```python
from build123d import *

# Parameters (mm, degrees)
F1_DEPTH = 30
F2_W     = 30
F2_H     = 30
F3_DEPTH = 1440
F4_W     = 1440
F4_H     = 1640
F5_DEPTH = 30
F7_DEPTH = 30


with BuildPart() as f1:
    # F0 (on Front) → F1 (new body)
    with BuildSketch(Plane.XZ):
        Polygon((0, 1700), (0, 0), (1500, 0), (1500, 1700), (0, 1900), align=None)
        Polygon((30, 1500), (30, 1670), (1470, 1670), (1470, 30), (30, 30), align=None, mode=Mode.SUBTRACT)
        Polygon((30, 1865.734508), (1273.008811, 1700), (30, 1700), align=None, mode=Mode.SUBTRACT)
    extrude(amount=F1_DEPTH)

    # F2 (on face) → F3 (join)
    with BuildSketch(Plane.XZ.offset(30)):
        with Locations((15, 15)):
            Rectangle(F2_W, F2_H)
        with Locations((1485, 15)):
            Rectangle(F2_W, F2_H)
        with Locations((15, 1685)):
            Rectangle(F2_W, F2_H)
        with Locations((1485, 1685)):
            Rectangle(F2_W, F2_H)
        with Locations((15, 1880.734508)):
            Rectangle(F2_W, F2_H)
        with Locations((750, 1787)):
            Rectangle(F2_W, F2_H)
    extrude(amount=F3_DEPTH)

    # F4 (on face) → F5 (join)
    with BuildSketch(Plane.XZ.offset(1470)):
        Polygon((0, 1900), (0, 0), (1500, 0), (1500, 1670), (1500, 1700), align=None)
        with Locations((750, 850)):
            Rectangle(F4_W, F4_H, mode=Mode.SUBTRACT)
        Polygon((30, 1700), (30, 1865.734508), (1273.008811, 1700), align=None, mode=Mode.SUBTRACT)
    extrude(amount=F5_DEPTH)

    # F6 (on face) → F7 (join)
    with BuildSketch(Plane.YZ.offset(1500)):
        Polygon((-1070, 1470), (-1070, 30), (-1040, 30), (-1040, 1470), (-460, 1470), (-460, 30), (-430, 30), (-430, 1470), (-30, 1470), (-30, 1500), (-1470, 1500), (-1470, 1470), align=None)
    extrude(amount=-F7_DEPTH)


solid = f1.part
```
Read the model definition and answer for the solid it produces. Units are mm, in the model's axes. A direction names the side the tool comes from. Coordinates: 2 decimals unless noted, no trailing zeros. Write each loop counter-clockwise with the first axis right and the second up, starting at its lowest first coordinate (ties: lowest second). Pieces come first, ordered by that corner, then holes. Notation, with made-up numbers: (4, 54.5) -> (42, 54.5) arc R19 cw to (42, 66.5) -> close; hole circle Ø4 at (-21.5, 30). An arc over 180 degrees is marked (long way). Answer as a JSON object with one key per item and string values.
Q1. Flat-ended cylindrical pins translate along their axes: pin 1 Ø15 at (y, z) = (-496.5, 1791.5) entering from +X; pin 2 Ø9 at (x, y) = (14, -1056) entering from +Z; pin 3 Ø24 at (x, y) = (1486, -839) entering from +Z. Find the tip coordinate at first contact, or state that the pin passes through.
The answers:
{"pin 1": "stops at x = 765", "pin 2": "stops at z = 1895.73", "pin 3": "stops at z = 1700"}
Q2. The part is cut by section D-D on x = 605. Give the vertices of the cut face in (y, z), then the cut area to 3 significant figures.
The answers:
{"outline": "(-1500, 0) -> (-1470, 0) -> (-1470, 30) -> (-1500, 30) -> close; (-1500, 1670) -> (-1470, 1670) -> (-1470, 1700) -> (-1500, 1700) -> close; (-1500, 1789.07) -> (-1470, 1789.07) -> (-1470, 1819.33) -> (-1500, 1819.33) -> close; (-30, 0) -> (0, 0) -> (0, 30) -> (-30, 30) -> close; (-30, 1670) -> (0, 1670) -> (0, 1700) -> (-30, 1700) -> close; (-30, 1789.07) -> (0, 1789.07) -> (0, 1819.33) -> (-30, 1819.33) -> close", "area": "5,420 mm2"}
Q3. The part is cut by section C-C on z = 419. Give the vertices of the cut face in (x, y).
The answers:
{"outline": "(0, -1500) -> (30, -1500) -> (30, -1470) -> (0, -1470) -> close; (0, -30) -> (30, -30) -> (30, 0) -> (0, 0) -> close; (1470, -1500) -> (1500, -1500) -> (1500, -1470) -> (1470, -1470) -> close; (1470, -1070) -> (1500, -1070) -> (1500, -1040) -> (1470, -1040) -> close; (1470, -460) -> (1500, -460) -> (1500, -430) -> (1470, -430) -> close; (1470, -30) -> (1500, -30) -> (1500, 0) -> (1470, 0) -> close"}
Q4. A tool of negligible diameter and unlimited length cuts with its end or side. For faces 4 (the flat face through (1470, -24, 460)), 5 (the flat face through (0, -24, 1377)), from which of +Z, -Z, +X, -X, +Y, -Y can it reach the whole face along a straight path? Write none if from no direction.
The answers:
{"face 4": "none", "face 5": "+Z, -Z, -X, +Y, -Y"}
Q5. Determine the mould class of faces 1 (the flat face through (24, 0, 1166)), 2 (the flat face through (643, -1485, 1784)), 3 (the flat face through (413, -24, 0)) for opening direction Z: pulls with the +Z half, pulls with the -Z half, needs draft (parallel to the pull), parting line crosses it, or undercut.
The answers:
{"face 1": "needs draft", "face 2": "undercut", "face 3": "pulls with the -Z half"}
Q6. The part is cut by section B-B on z = 1591.5. Give the vertices of the cut face in (x, y).
The answers:
{"outline": "(0, -1500) -> (30, -1500) -> (30, -1470) -> (0, -1470) -> close; (0, -30) -> (30, -30) -> (30, 0) -> (0, 0) -> close; (1470, -1500) -> (1500, -1500) -> (1500, -1470) -> (1470, -1470) -> close; (1470, -30) -> (1500, -30) -> (1500, 0) -> (1470, 0) -> close"}
Q7. Consider line 1 (X direction, y = -1422, z = 1671.5); line 2 (X direction, y = -221.5, z = 1786). Determine where each line is inside the solid, lowest interval first. Write a range as [from, to].
The answers:
{"line 1": "x = [0, 30], [1470, 1500]", "line 2": "x = [735, 765]"}
Q8. The part is cut by section A-A on y = -1105.5. Give the vertices of the cut face in (x, z).
The answers:
{"outline": "(0, 0) -> (30, 0) -> (30, 30) -> (0, 30) -> close; (0, 1670) -> (30, 1670) -> (30, 1700) -> (0, 1700) -> close; (0, 1865.73) -> (30, 1865.73) -> (30, 1895.73) -> (0, 1895.73) -> close; (735, 1772) -> (765, 1772) -> (765, 1802) -> (735, 1802) -> close; (1470, 0) -> (1500, 0) -> (1500, 30) -> (1470, 30) -> close; (1470, 1470) -> (1500, 1470) -> (1500, 1500) -> (1470, 1500) -> close; (1470, 1670) -> (1500, 1670) -> (1500, 1700) -> (1470, 1700) -> close"}
